Design review of the part built by this model. Coordinates are the model's own, in mm. A direction names the side the tool comes from. Round coordinates to 2 decimals unless told otherwise and drop trailing zeros. Loops run counter-clockwise (first coordinate to the right, second up) from the corner with the lowest first, then second, coordinate; pieces in that order, holes last. Notation, with made-up numbers: (74, 29) -> (133, 29) arc R11 ccw to (133, 42) -> close; hole circle Ø10 at (58.5, 11). An arc over 180 degrees is marked (long way). Answer as CSV lines item,"result". Start each with the question number.
(1) Take a section at D-D, the plane z = -45. Write out the cut boundary in (x, y), and give its area (3 significant figures).
(2) To check wall thickness, follow line 1 (Y direction, x = 54.9, z = -76); line 2 (X direction, y = -1.5, z = -36); line 3 (Z direction, x = 9, y = -0.75). State the ranges of each line that lie inside material, in increasing order. Write a range as from..to.
(3) Machinability: for faces 5 (the face through (3, -9, -5)), 6 (the face through (55, -3, -12)), 7 (the face through (6, -6, -5)), 8 (the face through (29, -2, -88)), which of the approach directions +Z, -Z, +X, -X, +Y, -Y give a long, thin tool a straight path to every point of the face, cutting with its end or side? Answer none if there is none.
(4) Draft analysis for pull direction Y (two halves, no side actions). For faces 1 (the face through (2.958, -5.369, -22.003)), 2 (the face through (55, -6, -23)), 3 (the face through (3.969, -7.863, -5.465)), 4 (the face through (55, -9, -5)), state which applies: +Y half, -Y half, draft (parallel to the pull), parting line (faces both ways), or undercut.
(5) Take a section at C-C, the plane y = -2. Write out the cut boundary in (x, z).
(6) For P1, Ø0.9, axis at x = 55.5, y = -5.5, coming from the +Z side; P2, Ø4, axis at y = -6, z = -20, coming from the -X side; P3, Ø1.8, axis at x = 2, z = -84, coming from the -Y side; P4, Ø1.8, axis at x = 54.5, y = -5, coming from the -Z side, all flat-tipped, find the tip position at first contact; note any pin that passes through.
(7) Take a section at B-B, the plane x = 3. State how many separate pieces and enclosed holes the cut face has, and give its area (3 significant figures).
(8) Take a section at A-A, the plane z = -76. Write out the cut boundary in (x, y).
from build123d import *

# Parameters (mm, degrees)
SKETCH1_R               = 2.1
BOSS_EXTRUDE1_DEPTH     = 6
FILLET1_R               = 1.5
SKETCH2_R               = 2.1
CUT_EXTRUDE1_DEPTH      = 5
CUT_EXTRUDE2_START      = -85
SKETCH2_2_R             = 2.1
CUT_EXTRUDE2_DEPTH      = 5
SKETCH4_W               = 23
SKETCH4_H               = 3
BOSS_EXTRUDE2_DEPTH     = 5
BOSS_EXTRUDE3_START     = -3
BOSS_EXTRUDE3_OUTLINE_W = 23
BOSS_EXTRUDE3_OUTLINE_H = 5
BOSS_EXTRUDE3_DEPTH     = 3


# Read off the part's stored shape, not the designer's step: Boss-Extrude3
with BuildPart() as part:
    # Sketch1 → Boss-Extrude1 (new body)
    with BuildSketch(Plane(origin=(0, 0, 0), x_dir=(0, 0, -1), z_dir=(1, 0, 0))):
        Polygon((84, 0), (3, 0), (3, -9), (8, -9), (8, -3), (17, -3), (17, -9), (23, -9), (23, -3), (73, -3), (73, -9), (79, -9), (79, -3), (88, -3), (88, -9), (93, -9), (93, 0), align=None)
        with Locations((20, -6)):
            Circle(SKETCH1_R, mode=Mode.SUBTRACT)
        with Locations((76, -6)):
            Circle(SKETCH1_R, mode=Mode.SUBTRACT)
    extrude(amount=BOSS_EXTRUDE1_DEPTH)

    # Fillet1
    fillet1_edges = [part.edges().sort_by_distance(p)[0] for p in [
        (3, -9, -23),
        (3, -9, -17),
        (3, -3, -17),
        (3, -3, -79),
        (3, -9, -79),
        (3, -9, -73),
        (3, -3, -73),
        (3, -3, -23),
    ]]
    fillet(fillet1_edges, radius=FILLET1_R)

    # Sketch2 → Cut-Extrude1 (cut)
    with BuildSketch(Plane.XY.offset(-3)):
        with Locations((3, -6)):
            Circle(SKETCH2_R)
    extrude(amount=-CUT_EXTRUDE1_DEPTH, mode=Mode.SUBTRACT)

    # Sketch2<2> → Cut-Extrude2 (cut)
    with BuildSketch(Plane.XY.offset(-3).offset(CUT_EXTRUDE2_START)):
        with Locations((3, -6)):
            Circle(SKETCH2_2_R)
    extrude(amount=-CUT_EXTRUDE2_DEPTH, mode=Mode.SUBTRACT)

    # Sketch4 → Boss-Extrude2 (add)
    with BuildSketch(Plane.XY.offset(-3)):
        with Locations((17.5, -1.5)):
            Rectangle(SKETCH4_W, SKETCH4_H)
    extrude(amount=-BOSS_EXTRUDE2_DEPTH)

    # Boss-Extrude3 outline → Boss-Extrude3 (add)
    with BuildSketch(Plane(origin=(0, 0, 0), x_dir=(1, 0, 0), z_dir=(0, 1, 0)).offset(BOSS_EXTRUDE3_START)):
        with Locations((17.5, 90.5)):
            Rectangle(BOSS_EXTRUDE3_OUTLINE_W, BOSS_EXTRUDE3_OUTLINE_H)
    extrude(amount=BOSS_EXTRUDE3_DEPTH)

    # Mirror1: part across plane


with BuildPart() as part_1:
    add(part.part)
    add(part.part.mirror(Plane(origin=(29, 0, 0), x_dir=(0, 0, 1), z_dir=(1, 0, 0))))


solid = part_1.part
The answers:
1,outline,"(0, -3) -> (6, -3) -> (6, 0) -> (0, 0) -> close; (52, -3) -> (58, -3) -> (58, 0) -> (52, 0) -> close"
1,area,"36.0 mm²"
2,line 1,"-9..-8.1, -3.9..0"
2,line 2,"0..6, 52..58"
2,line 3,"-93..-88, -8..-3"
3,face 5,"+Z, -Z, +X, -X, -Y"
3,face 6,"+X, -X, -Y"
3,face 7,"+Z, -Z, -Y"
3,face 8,"+Y, -Y"
4,face 1,"undercut"
4,face 2,"draft"
4,face 3,"undercut"
4,face 4,"-Y half"
5,outline,"(0, -93) -> (58, -93) -> (58, -3) -> (0, -3) -> close; hole (6, -88) -> (52, -88) -> (52, -8) -> (6, -8) -> close"
6,P1,"z = -17"
6,P2,"through"
6,P3,"y = -3"
6,P4,"z = -79.05"
7,separate pieces,"3"
7,enclosed holes,"2"
7,area,"332 mm²"
8,outline,"(0, -9) -> (6, -9) -> (6, -8.1) -> (0, -8.1) -> close; (0, -3.9) -> (6, -3.9) -> (6, 0) -> (0, 0) -> close; (52, -9) -> (58, -9) -> (58, -8.1) -> (52, -8.1) -> close; (52, -3.9) -> (58, -3.9) -> (58, 0) -> (52, 0) -> close"
